Read the model definition and answer for the solid it produces. Units are mm, in the model's axes. Coordinates: 2 decimals unless noted, no trailing zeros. Loops run counter-clockwise (first coordinate to the right, second up) from the corner with the lowest first, then second, coordinate; pieces in that order, holes last. Notation, with made-up numbers: (21.5, -29.75) - (48.5, -29.75) arc R19 ccw to (48.5, -25.75) - close; hole circle Ø6 at (53.25, 5.25). An arc over 180 degrees is marked (long way). One line per question, with ' | ' between items. Start each with the question number.
```python
from build123d import *

# Parameters (mm, degrees)
BOSS_EXTRUDE1_DEPTH = 5
SKETCH3_R           = 9
BOSS_EXTRUDE2_DEPTH = 15
SKETCH5_R           = 5
CUT_EXTRUDE1_DEPTH  = 15


with BuildPart() as part:
    # Sketch1 → Boss-Extrude1 (new body)
    with BuildSketch(Plane(origin=(0, 0, 0), x_dir=(1, 0, 0), z_dir=(0, 1, 0))):
        Polygon((-50, 10), (50, 10), (80, 0), (50, -10), (-50, -10), (-80, 0), align=None)
    extrude(amount=BOSS_EXTRUDE1_DEPTH)

    # Sketch3 → Boss-Extrude2 (add)
    with BuildSketch(Plane(origin=(0, 5, 0), x_dir=(1, 0, 0), z_dir=(0, 1, 0))):
        with Locations(Location((0, 0, 0), (0, 0, 270))):
            Circle(SKETCH3_R)
    extrude(amount=BOSS_EXTRUDE2_DEPTH)

    # Sketch5 → Cut-Extrude1 (cut)
    with BuildSketch(Plane(origin=(0, 5, 0), x_dir=(1, 0, 0), z_dir=(0, 1, 0))):
        with Locations(Location((60, 0, 0), (0, 0, 270))):
            Circle(SKETCH5_R)
        with Locations(Location((-60, 0, 0), (0, 0, 270))):
            Circle(SKETCH5_R)
    extrude(amount=-CUT_EXTRUDE1_DEPTH, mode=Mode.SUBTRACT)


solid = part.part
```
1) The part is cut by section D-D on z = -7.25. Write down the section's boundary in (x, y).
2) The mould has two halves that part along Z. Classify faces 1 (the flat face through (-65, 2, 5)), 2 (the cylindrical face through (2.703, 12.395, 8.584)), 3 (the cylindrical face through (-55.043, 2.535, -0.651)), 4 (the cylindrical face through (64, 3, 3)): released by +Z, released by -Z, zero draft, split by the parting line, or undercut.
3) The part is cut by section A-A on x = -60. Write down the section's boundary in (y, z).
4) The part is cut by section B-B on x = 0. Write down the section's boundary in (y, z), and give its area (3 significant figures).
5) Given pin 1 Ø2 at (x, z) = (-43.5, 6) entering from +Y; pin 2 Ø8 at (x, z) = (60, 0) entering from -Y; pin 3 Ø12 at (y, z) = (15, 4) entering from +X, each flat-ended and moving along its own axis, determine where each tip first touches the part or whether it passes through.
6) Find the intervals of material crossed by line 1 along Y through (x, z) = (19, 8.25); line 2 along X through (y, z) = (19, 7); line 3 along X through (y, z) = (17.75, 5.25), in increasing order. Write a range as from..to.
7) The part is cut by section C-C on y = 6.75. Write down the section's boundary in (x, z), and give its area (3 significant figures).
Answer below:
1) outline: (-58.25, 0) - (58.25, 0) - (58.25, 5) - (5.33, 5) - (5.33, 20) - (-5.33, 20) - (-5.33, 5) - (-58.25, 5) - close
2) face 1: released by +Z | face 2: split by the parting line | face 3: undercut | face 4: undercut
3) outline: (0, -6.67) - (5, -6.67) - (5, -5) - (0, -5) - close; (0, 5) - (5, 5) - (5, 6.67) - (0, 6.67) - close
4) outline: (0, -10) - (5, -10) - (5, -9) - (20, -9) - (20, 9) - (5, 9) - (5, 10) - (0, 10) - close | area: 370 mm2
5) pin 1: y = 5 | pin 2: through | pin 3: x = 9
6) line 1: 0..5 | line 2: -5.66..5.66 | line 3: -7.31..7.31
7) outline: circle Ø18 at (0, 0) | area: 254 mm2
